```python
from build123d import *

# Parameters (mm, degrees)
ESQUISSE1_R             = 22.5
BOSS_EXTRU_1_DEPTH      = 5
ESQUISSE6_R             = 2.55
ENL_V_MAT_EXTRU_4_DEPTH = 5
ESQUISSE7_R             = 18.80314531
ESQUISSE7_R_2           = 16.53251654
ENL_V_MAT_EXTRU_5_DEPTH = 1


with BuildPart() as part:
    # Esquisse1 → Boss.-Extru.1 (new body)
    with BuildSketch(Plane.XY):
        Circle(ESQUISSE1_R)
    extrude(amount=BOSS_EXTRU_1_DEPTH)

    # Esquisse6 → Enlèv. mat.-Extru.4 (cut)
    with BuildSketch(Plane.XY.offset(5)):
        Circle(ESQUISSE6_R)
    extrude(amount=-ENL_V_MAT_EXTRU_4_DEPTH, mode=Mode.SUBTRACT)

    # Esquisse7 → Enlèv. mat.-Extru.5 (cut)
    with BuildSketch(Plane.XY.offset(5)):
        Circle(ESQUISSE7_R)
        Circle(ESQUISSE7_R_2, mode=Mode.SUBTRACT)
    extrude(amount=-ENL_V_MAT_EXTRU_5_DEPTH, mode=Mode.SUBTRACT)


solid = part.part
```
Input: part model. Units: mm. Frame: model coordinates. A direction names the side the tool comes from. Coordinates: 2 decimals unless noted, no trailing zeros. Loops run counter-clockwise (first coordinate to the right, second up) from the corner with the lowest first, then second, coordinate; pieces in that order, holes last. Notation, with made-up numbers: M 4,-19 L 53,-19 A27 cw 53,-2 Z; hole C 63.5,-25.5 d4. An arc over 180 degrees is marked long. Answer in a Markdown table with one row per item.
1. Draft query along X for faces 1 (the flat face through (0, -3, 5)), 2 (the flat face through (0, -17, 4)), 3 (the cylindrical face through (10.382, -19.961, 2.465)). Return one class per face: pulls with the +X half, pulls with the -X half, needs draft (parallel to the pull), parting line crosses it, or undercut.
Response:
| item | result |
|---|---|
| face 1 | needs draft |
| face 2 | undercut |
| face 3 | parting line crosses it |
2. Reachability of faces 4 (the cylindrical face through (-2.448, 18.643, 4.507)), 5 (the cylindrical face through (1.18, -2.26, 2.54)) from +Z, -Z, +X, -X, +Y, -Y: full face, straight path, thin tool, end or side. Return the list, or none.
Response:
| item | result |
|---|---|
| face 4 | +Z |
| face 5 | +Z, -Z |
3. Section D-D, the plane z = 2.7. Output: boundary loops of the cut face in (x, y), then the cut area to 3 significant figures.
Response:
| item | result |
|---|---|
| outline | C 0,0 d45; hole C 0,0 d5.1 |
| area | 1,570 mm2 |
4. First-contact query: pin 1 (1 mm diameter, centred on y = -7.5, z = 2.5, fed in from -X); pin 2 (10 mm diameter, centred on x = -13.5, y = 9.5, fed in from -Z); pin 3 (1 mm diameter, centred on x = -4.5, z = 3, fed in from +Y). Flat tips, straight axial feed; report the tip coordinate or a pass-through.
Response:
| item | result |
|---|---|
| pin 1 | stops at x = -21.38 |
| pin 2 | stops at z = 0 |
| pin 3 | stops at y = 22.14 |
5. Section A-A, the plane y = 0. Output: boundary loops of the cut face in (x, z), then the cut area to 3 significant figures.
Response:
| item | result |
|---|---|
| outline | M -22.5,0 L -2.55,0 L -2.55,5 L -16.53,5 L -16.53,4 L -18.8,4 L -18.8,5 L -22.5,5 Z; M 2.55,0 L 22.5,0 L 22.5,5 L 18.8,5 L 18.8,4 L 16.53,4 L 16.53,5 L 2.55,5 Z |
| area | 195 mm2 |
6. Material intervals for line 1 (Y direction, x = 0, z = 4.45); line 2 (Y direction, x = 0, z = 2.05); line 3 (Y direction, x = 1.5, z = 3.1), sorted ascending.
Response:
| item | result |
|---|---|
| line 1 | y = -22.5 to -18.8, -16.53 to -2.55, 2.55 to 16.53, 18.8 to 22.5 |
| line 2 | y = -22.5 to -2.55, 2.55 to 22.5 |
| line 3 | y = -22.45 to -2.06, 2.06 to 22.45 |
7. Section C-C, the plane x = 4.5. Output: boundary loops of the cut face in (y, z), then the cut area to 3 significant figures.
Response:
| item | result |
|---|---|
| outline | M -22.05,0 L 22.05,0 L 22.05,5 L 18.26,5 L 18.26,4 L 15.91,4 L 15.91,5 L -15.91,5 L -15.91,4 L -18.26,4 L -18.26,5 L -22.05,5 Z |
| area | 216 mm2 |
